from build123d import *

# Parameters (mm, degrees)
SKETCH1_R                 = 1.5
BOSS_EXTRUDE1_DEPTH       = 3
BOSS_EXTRUDE2_START       = 22.5
SKETCH2_W                 = 1.6
SKETCH2_H                 = 6
BOSS_EXTRUDE2_DEPTH       = 29
SKETCH4_R                 = 1.5
BOSS_EXTRUDE5_DEPTH       = 1
CHAMFER2_SIZE             = 2
CHAMFER2_SIZE2            = 3.464101615
SKETCH3_W                 = 24
SKETCH3_H                 = 29
SKETCH3_R                 = 11
BOSS_EXTRUDE4_DEPTH       = 7
CHAMFER3_SIZE             = 2
CHAMFER2_OF_MIRROR1_SIZE2 = 2
CHAMFER2_OF_MIRROR1_SIZE  = 3.464101615
SKETCH5_R                 = 2
BOSS_EXTRUDE6_DEPTH       = 14
CHAMFER5_SIZE             = 5


with BuildPart() as part:
    # Sketch1 → Boss-Extrude1 (new body)
    with BuildSketch(Plane(origin=(0, 0, 0), x_dir=(1, 0, 0), z_dir=(0, 1, 0))):
        Polygon((-6, 17), (-3, 20), (3, 20), (6, 17), (6, -17), (3, -20), (-3, -20), (-6, -17), align=None)
        with Locations(Location((0, 14, 0), (0, 0, 270))):
            Circle(SKETCH1_R, mode=Mode.SUBTRACT)
        with Locations(Location((0, -14, 0), (0, 0, 270))):
            Circle(SKETCH1_R, mode=Mode.SUBTRACT)
    boss_extrude1 = extrude(amount=BOSS_EXTRUDE1_DEPTH)

    # Sketch2 → Boss-Extrude2 (add)
    with BuildSketch(Plane(origin=(0, 3, 0), x_dir=(1, 0, 0), z_dir=(0, 1, 0)).offset(BOSS_EXTRUDE2_START)):
        with Locations((-5.3, 9)):
            Rectangle(SKETCH2_W, SKETCH2_H)
        with Locations((-5.3, -9)):
            Rectangle(SKETCH2_W, SKETCH2_H)
    extrude(amount=-BOSS_EXTRUDE2_DEPTH)

    # Sketch4 → Boss-Extrude5 (add)
    with BuildSketch(Plane(origin=(0, 3, 0), x_dir=(1, 0, 0), z_dir=(0, 1, 0))):
        Polygon((-3, 20), (-6, 17), (-6, 12), (-4.5, 12), (-4.5, 6), (-6, 6), (-6, -6), (-4.5, -6), (-4.5, -12), (-6, -12), (-6, -17), (-3, -20), (3, -20), (6, -17), (6, 17), (3, 20), align=None)
        with Locations(Location((0, 14, 0), (0, 0, 270))):
            Circle(SKETCH4_R, mode=Mode.SUBTRACT)
        with Locations(Location((0, -14, 0), (0, 0, 270))):
            Circle(SKETCH4_R, mode=Mode.SUBTRACT)
    boss_extrude5 = extrude(amount=BOSS_EXTRUDE5_DEPTH)

    # Chamfer2
    chamfer2_edges = [part.edges().sort_by_distance(p)[0] for p in [
        (-4.5, 0, 9),
        (-4.5, 0, -9),
    ]]
    chamfer2_side = [part.faces().sort_by_distance(p)[0] for p in [
        (0.219837568, 0, 0),
    ]]
    chamfer(chamfer2_edges, length=CHAMFER2_SIZE, length2=CHAMFER2_SIZE2, reference=chamfer2_side[0])

    # Sketch3 → Boss-Extrude4 (add)
    with BuildSketch(Plane.ZY.offset(6.1)):
        with Locations((0, 11)):
            Rectangle(SKETCH3_W, SKETCH3_H)
        with Locations(Location((0, 11, 0), (0, 0, 236.944268849))):
            Circle(SKETCH3_R, mode=Mode.SUBTRACT)
    extrude(amount=BOSS_EXTRUDE4_DEPTH)

    # Chamfer3
    chamfer3_edges = [part.edges().sort_by_distance(p)[0] for p in [
        (-8.8, 25.5, -12),
        (-8.8, -3.5, -12),
        (-8.8, -3.5, 12),
        (-8.8, 25.5, 12),
    ]]
    chamfer(chamfer3_edges, length=CHAMFER3_SIZE)

    # Mirror1: Boss-Extrude1, Boss-Extrude5 across plane
    add(boss_extrude1.mirror(Plane(origin=(0, 11, 0), x_dir=(0, 0, 1), z_dir=(0, -1, 0))))
    add(boss_extrude5.mirror(Plane(origin=(0, 11, 0), x_dir=(0, 0, 1), z_dir=(0, -1, 0))))

    # Chamfer2 of Mirror1
    chamfer2_of_mirror1_edges = [part.edges().sort_by_distance(p)[0] for p in [
        (-4.5, 22, 9),
        (-4.5, 22, -9),
    ]]
    chamfer(chamfer2_of_mirror1_edges, length=CHAMFER2_OF_MIRROR1_SIZE, length2=CHAMFER2_OF_MIRROR1_SIZE2)

    # Sketch5 → Boss-Extrude6 (add)
    # profile 1 of 2: a face of its own
    with BuildSketch(Plane(origin=(0, 4, 0), x_dir=(1, 0, 0), z_dir=(0, 1, 0))):
        Polygon((6, -6), (-6, -6), (-6, -17), (-3, -20), (3, -20), (6, -17), align=None)
        with Locations(Location((0, -14, 0), (0, 0, 90))):
            Circle(SKETCH5_R, mode=Mode.SUBTRACT)
    # profile 2 of 2: a face of its own
    with BuildSketch(Plane(origin=(0, 4, 0), x_dir=(1, 0, 0), z_dir=(0, 1, 0))):
        Polygon((-6, 17), (-6, 6), (6, 6), (6, 17), (3, 20), (-3, 20), align=None)
        with Locations(Location((0, 14, 0), (0, 0, 90))):
            Circle(SKETCH5_R, mode=Mode.SUBTRACT)
    extrude(amount=BOSS_EXTRUDE6_DEPTH)

    # Chamfer5
    chamfer5_edges = [part.edges().sort_by_distance(p)[0] for p in [
        (-6, 11, 12),
        (-6, 11, -12),
    ]]
    chamfer(chamfer5_edges, length=CHAMFER5_SIZE - 0.0001)  # a hair under: the kernel refuses the full size


solid = part.part
Model file for the job. Use its own axes, mm. A direction names the side the tool comes from. Coordinates: 2 decimals unless noted, no trailing zeros. Order: outer loops, then holes, each group sorted by start corner. A loop starts at its lowest first (then second) coordinate and runs counter-clockwise, first axis right, second up. Notation, with made-up numbers: M -38.5,18.5 L 16.5,18.5 A36 cw 16.5,54.5 Z; hole C 7.5,-36 d8. An arc over 180 degrees is marked long. Return JSON: item names as keys, results as strings.
1. Saw through at A-A (y = 11). Give the number of separate pieces and of enclosed holes in the cut face, and give its area (3 significant figures).
Ans:
{"separate pieces": "2", "enclosed holes": "2", "area": "333 mm^2"}
2. Saw through at D-D (z = -13). Give the cut face in (x, y), and give its area (3 significant figures).
Ans:
{"outline": "M -10,0 L -1.12,0 L -1.12,4 L -1.73,4 L -1.73,18 L -1.12,18 L -1.12,22 L -10,22 Z; M 1.12,0 L 6,0 L 6,22 L 1.12,22 L 1.12,18 L 1.73,18 L 1.73,4 L 1.12,4 Z", "area": "286 mm^2"}
3. Drill centre lines: probe 1 along Y at (x, z) = (3, -4.5); probe 2 along Z at (x, y) = (-0.5, 16.25); probe 3 along Z at (x, y) = (-1.5, 4.25). Where is each one in solid material? Low to high.
Ans:
{"probe 1": "0 to 4, 18 to 22", "probe 2": "-20 to -15.94, -12.06 to -6, 6 to 12.06, 15.94 to 20", "probe 3": "-20 to -15.32, -12.68 to -6, 6 to 12.68, 15.32 to 20"}
4. Tool access for faces 1 (the face through (-9.551, 0.404, -2.954)), 2 (the face through (-12, 11, -12)), 3 (the face through (0, 22, 0)), 4 (the face through (-6.1, 23, 0)): list every direction of +Z, -Z, +X, -X, +Y, -Y with a clear straight run to the whole face (end or side of a thin tool).
Ans:
{"face 1": "-X", "face 2": "-Z, -X", "face 3": "+X, +Y", "face 4": "+Y, -Y"}
5. Saw through at C-C (z = 0). Give the cut face in (x, y), and give its area (3 significant figures).
Ans:
{"outline": "M -13.1,-3.5 L -6.1,-3.5 L -6.1,0 L -13.1,0 Z; M -13.1,22 L -6.1,22 L -6.1,25.5 L -13.1,25.5 Z; M -6,0 L 6,0 L 6,4 L -6,4 Z; M -6,18 L 6,18 L 6,22 L -6,22 Z", "area": "145 mm^2"}
6. Pull direction X, two halves, no side cores. Call faces 5 (the face through (-6.1, 11, 8)), 6 (the face through (0, 18, 0)), 7 (the face through (6, 3.5, 0.2)), 8 (the face through (0.07, 1.97, 12.5)): +X half, -X half, draft (parallel to the pull), parting line (faces both ways), or undercut.
Ans:
{"face 5": "-X half", "face 6": "draft", "face 7": "+X half", "face 8": "undercut"}
7. Flat gauge pins, fed straight in: pin 1 (10 mm diameter, centred on x = -5, y = 0.5, fed in from -Z); pin 2 (4.5 mm diameter, centred on x = -1, z = 13.5, fed in from +Y); pin 3 (6 mm diameter, centred on y = 19.5, z = 15.5, fed in from -X); pin 4 (4 mm diameter, centred on x = 0, z = -14, fed in from -Y). Where does each tip first touch, or does it go through?
Ans:
{"pin 1": "z = -20", "pin 2": "y = 22.31", "pin 3": "x = -10.5", "pin 4": "y = 0"}
